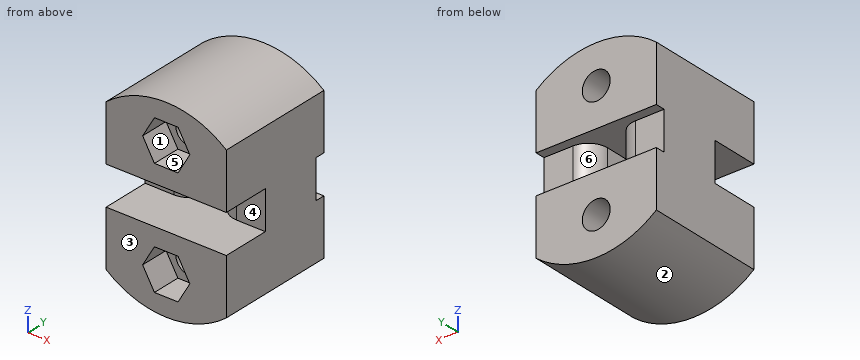
```python
from build123d import *

# Parameters (mm, degrees)
SKETCH1_R               = 20
BOSS_EXTRUDE1_DEPTH     = 25
SKETCH2_W               = 40
SKETCH2_H               = 8
CUT_EXTRUDE1_DEPTH      = 2
M5_CLEARANCE_HOLE1_D    = 5.8
CUT_EXTRUDE2_DEPTH      = 6
CUT_EXTRUDE3_DEPTH      = 37.455452267
CUT_EXTRUDE3_DEPTH_BACK = 37.455452267
SKETCH6_W               = 5
SKETCH6_H               = 8
SKETCH7_W               = 40
SKETCH7_H               = 8
CUT_EXTRUDE4_DEPTH      = 10
FILLET1_R               = 4
SKETCH8_OUTSIDE_W       = 54.37
SKETCH8_OUTSIDE_H       = 54.37
SKETCH8_OUTSIDE_W_2     = 25
SKETCH8_OUTSIDE_H_2     = 40
CUT_EXTRUDE5_DEPTH      = 38.749172176


with BuildPart() as part:
    # Sketch1 → Boss-Extrude1 (new body)
    with BuildSketch(Plane(origin=(0, 0, 0), x_dir=(1, 0, 0), z_dir=(0, 1, 0))):
        with Locations(Location((0, 0, 0), (0, 0, 270))):
            Circle(SKETCH1_R)
    extrude(amount=BOSS_EXTRUDE1_DEPTH)

    # Sketch2 → Cut-Extrude1 (cut)
    with BuildSketch(Plane(origin=(0, 25, 0), x_dir=(1, 0, 0), z_dir=(0, 1, 0))):
        Rectangle(SKETCH2_W, SKETCH2_H)
    extrude(amount=-CUT_EXTRUDE1_DEPTH, mode=Mode.SUBTRACT)

    # M5 Clearance Hole1 (through all)
    with Locations(Plane(origin=(0, 25, -12), x_dir=(0, 0, 1), z_dir=(0, 1, 0))):
        with Locations((0, 0), (24, 0)):
            Hole(M5_CLEARANCE_HOLE1_D / 2)

    # Sketch5 → Cut-Extrude2 (cut)
    with BuildSketch(Plane.XZ):
        Polygon((4.907477288, 12), (2.453738644, 16.25), (-2.453738644, 16.25), (-4.907477288, 12), (-2.453738644, 7.75), (2.453738644, 7.75), align=None)
        Polygon((4.907477288, -12), (2.453738644, -7.75), (-2.453738644, -7.75), (-4.907477288, -12), (-2.453738644, -16.25), (2.453738644, -16.25), align=None)
    extrude(amount=-CUT_EXTRUDE2_DEPTH, mode=Mode.SUBTRACT)

    # Sketch6 → Cut-Extrude3 (cut, two sides: drawn at the far end of the back side and taken through both)
    with BuildSketch(Plane(origin=(0, 23, 0), x_dir=(1, 0, 0), z_dir=(0, 1, 0)).offset(-CUT_EXTRUDE3_DEPTH_BACK)):
        Rectangle(SKETCH6_W, SKETCH6_H)
    extrude(amount=CUT_EXTRUDE3_DEPTH + CUT_EXTRUDE3_DEPTH_BACK, mode=Mode.SUBTRACT)

    # Sketch7 → Cut-Extrude4 (cut)
    with BuildSketch(Plane.XZ):
        Rectangle(SKETCH7_W, SKETCH7_H)
    extrude(amount=-CUT_EXTRUDE4_DEPTH, mode=Mode.SUBTRACT)

    # Fillet1
    fillet1_edges = [part.edges().sort_by_distance(p)[0] for p in [
        (2.5, 10, 0),
        (-2.5, 10, 0),
        (-2.5, 23, 0),
        (2.5, 23, 0),
    ]]
    fillet(fillet1_edges, radius=FILLET1_R)

    # Sketch8 outside → Cut-Extrude5 (cut, through all)
    with BuildSketch(Plane(origin=(0, 25, 0), x_dir=(1, 0, 0), z_dir=(0, 1, 0))):
        Rectangle(SKETCH8_OUTSIDE_W, SKETCH8_OUTSIDE_H)
        Rectangle(SKETCH8_OUTSIDE_W_2, SKETCH8_OUTSIDE_H_2, mode=Mode.SUBTRACT)
    extrude(amount=-CUT_EXTRUDE5_DEPTH, mode=Mode.SUBTRACT)


solid = part.part
```
Input: part model. Units: mm. Frame: model coordinates. Face numbers are marked on the shaded views. A direction names the side the tool comes from. Give positions to 0.01 mm unless a question says otherwise; leave off trailing zeros. Order: outer loops, then holes, each group sorted by start corner. A loop starts at its lowest first (then second) coordinate and runs counter-clockwise, first axis right, second up. Notation, with made-up numbers: (52.5, 80) -> (69.5, 80) arc R25 ccw to (69.5, 94) -> close; hole circle Ø1 at (18.25, -31.5). An arc over 180 degrees is marked (long way). Write each question's results on one line, items separated by ' | '. Start each with the question number.
Item 1: Line query: line 1 (X direction, y = 15, z = -12); line 2 (Z direction, x = 1.25, y = 17); line 3 (X direction, y = 21.75, z = -10). Output: solid intervals per line, ascending.
Item 2: Cut plane D-D on z = 13. Return the cut outline in (x, y), then the cut area to 3 significant figures.
Item 3: Cut plane A-A on y = 4.5. Return the cut outline in (x, z).
Item 4: Mould query, pull axis X, two halves, no side actions, for the marked faces 1, 2 and 3. Classes: pulls with the +X half, pulls with the -X half, needs draft (parallel to the pull), parting line crosses it, or undercut.
Item 5: Set-up query: the marked faces 4, 5 and 6. Return all of +Z, -Z, +X, -X, +Y, -Y with unobstructed straight access to the full face (end or side cutting, diameter ignored); none if empty.
Item 6: Cut plane C-C on y = 8.75. Return the cut outline in (x, z), then the cut area to 3 significant figures.
Item 7: Contact query for flat-ended pins moving along their axis: P1, Ø2.5, axis at x = -2, z = -12.5, coming from the -Y side; P2, Ø4, axis at x = -5, y = 13.5, coming from the +Z side; P3, Ø3, axis at x = 8.5, z = 0.5, coming from the -Y side. Output: stop coordinate, or through.
Item 8: Cut plane B-B on x = 0. Return the cut outline in (y, z), then the cut area to 3 significant figures.
Established:
1) line 1: -12.5 to -2.9, 2.9 to 12.5 | line 2: -19.96 to -14.62, -9.38 to -4, 4 to 9.38, 14.62 to 19.96 | line 3: -12.5 to -2.1, 2.1 to 12.5
2) outline: (-12.5, 0) -> (-4.33, 0) -> (-4.33, 6) -> (-2.72, 6) -> (-2.72, 25) -> (-12.5, 25) -> close; (2.72, 6) -> (4.33, 6) -> (4.33, 0) -> (12.5, 0) -> (12.5, 25) -> (2.72, 25) -> close | area: 470 mm^2
3) outline: (-12.5, -15.61) arc R20 ccw to (12.5, -15.61) -> (12.5, -4) -> (-12.5, -4) -> close; (-12.5, 4) -> (12.5, 4) -> (12.5, 15.61) arc R20 ccw to (-12.5, 15.61) -> close; hole (-4.91, -12) -> (-2.45, -16.25) -> (2.45, -16.25) -> (4.91, -12) -> (2.45, -7.75) -> (-2.45, -7.75) -> close; hole (-4.91, 12) -> (-2.45, 7.75) -> (2.45, 7.75) -> (4.91, 12) -> (2.45, 16.25) -> (-2.45, 16.25) -> close
4) face 1: undercut | face 2: parting line crosses it | face 3: needs draft
5) face 4: +X, -X, -Y | face 5: -Y | face 6: +Y
6) outline: (-12.5, -15.61) arc R20 ccw to (12.5, -15.61) -> (12.5, -4) -> (-12.5, -4) -> close; (-12.5, 4) -> (12.5, 4) -> (12.5, 15.61) arc R20 ccw to (-12.5, 15.61) -> close; hole circle Ø5.8 at (0, -12); hole circle Ø5.8 at (0, 12) | area: 678 mm^2
7) P1: y = 6 | P2: z = 19.77 | P3: y = 10
8) outline: (0, -20) -> (25, -20) -> (25, -14.9) -> (6, -14.9) -> (6, -16.25) -> (0, -16.25) -> close; (0, -7.75) -> (6, -7.75) -> (6, -9.1) -> (25, -9.1) -> (25, -4) -> (0, -4) -> close; (0, 4) -> (25, 4) -> (25, 9.1) -> (6, 9.1) -> (6, 7.75) -> (0, 7.75) -> close; (0, 16.25) -> (6, 16.25) -> (6, 14.9) -> (25, 14.9) -> (25, 20) -> (0, 20) -> close | area: 478 mm^2
